Read the model definition and answer for the solid it produces. Units are mm, in the model's axes. A direction names the side the tool comes from. Round coordinates to 2 decimals unless told otherwise and drop trailing zeros. Loops run counter-clockwise (first coordinate to the right, second up) from the corner with the lowest first, then second, coordinate; pieces in that order, holes last. Notation, with made-up numbers: (3.5, -2) -> (13.5, -2) arc R21 ccw to (13.5, 21) -> close; hole circle Ø10 at (57.5, -0.5). An arc over 180 degrees is marked (long way). Put each result on its own line as item: value.
from build123d import *

# Parameters (mm, degrees)
SKETCH_1_R          = 0.9
SKETCH_1_R_2        = 0.8
EXTRUDE_1_DEPTH     = 3.2
EXTRUDE_1_2_DEPTH   = 3.2
SKETCH_2_W          = 51.115590172
SKETCH_2_H          = 4.08
EXTRUDE_2_DEPTH     = 1.2
EXTRUDE_START       = -3.2
EXTRUDE_3_DEPTH     = 3.2
SKETCH_4_R          = 2
CUT_EXTRUDE_1_DEPTH = 2
FILLET_1_R          = 0.5


with BuildPart() as part:
    # Sketch 1 → Extrude 1 (new body)
    with BuildSketch(Plane.XY):
        with BuildLine():
            Line((-32.44, 5.005), (-31.75, 5.005))
            ThreePointArc((-31.75, 5.005), (-31.624500996, 4.977488532), (-31.522019738, 4.9))
            Line((-31.522019738, 4.9), (-28, 4.9))
            Line((-28, 4.9), (-28, 6.996662954))
            ThreePointArc((-28, 6.996662954), (-27.853553391, 7.350216345), (-27.5, 7.496662954))
            Line((-27.5, 7.496662954), (-22.181386307, 7.496662954))
            Line((-22.181386307, 7.496662954), (-22.181386307, 9.626936565))
            ThreePointArc((-22.181386307, 9.626936565), (-22.687871835, 9.843944297), (-23.142051903, 10.155938547))
            Line((-23.142051903, 10.155938547), (-24.268653026, 11.105751817))
            ThreePointArc((-24.268653026, 11.105751817), (-24.871565433, 11.455249887), (-25.557795086, 11.576662954))
            Line((-25.557795086, 11.576662954), (-30.347104952, 11.576662954))
            ThreePointArc((-30.347104952, 11.576662954), (-31.033334605, 11.455249887), (-31.636247011, 11.105751817))
            Line((-31.636247011, 11.105751817), (-32.42914206, 10.437278989))
            ThreePointArc((-32.42914206, 10.437278989), (-32.9535992, 9.751314044), (-33.14, 8.908190127))
            Line((-33.14, 8.908190127), (-33.14, 5.705))
            ThreePointArc((-33.14, 5.705), (-32.934974747, 5.210025253), (-32.44, 5.005))
        make_face()
        with Locations(Location((-27.952450019, 9.676662954, 0), (0, 0, 270))):
            Circle(SKETCH_1_R, mode=Mode.SUBTRACT)
        with Locations(Location((-31.24, 6.905, 0), (0, 0, 270))):
            Circle(SKETCH_1_R_2, mode=Mode.SUBTRACT)
    extrude(amount=EXTRUDE_1_DEPTH)



with BuildPart() as body_2:
    # Sketch 1 → Extrude 1 2 (new body)
    with BuildSketch(Plane.XY):
        with BuildLine():
            Line((28, 6.996662954), (28, 4.9))
            Line((28, 4.9), (31.522019738, 4.9))
            ThreePointArc((31.522019738, 4.9), (31.624500996, 4.977488532), (31.75, 5.005))
            Line((31.75, 5.005), (32.44, 5.005))
            ThreePointArc((32.44, 5.005), (32.934974747, 5.210025253), (33.14, 5.705))
            Line((33.14, 5.705), (33.14, 8.908190127))
            ThreePointArc((33.14, 8.908190127), (32.9535992, 9.751314044), (32.42914206, 10.437278989))
            Line((32.42914206, 10.437278989), (31.636247011, 11.105751817))
            ThreePointArc((31.636247011, 11.105751817), (31.033334605, 11.455249887), (30.347104952, 11.576662954))
            Line((30.347104952, 11.576662954), (25.557795086, 11.576662954))
            ThreePointArc((25.557795086, 11.576662954), (24.871565433, 11.455249887), (24.268653026, 11.105751817))
            Line((24.268653026, 11.105751817), (23.142051903, 10.155938547))
            ThreePointArc((23.142051903, 10.155938547), (22.687871835, 9.843944297), (22.181386307, 9.626936565))
            Line((22.181386307, 9.626936565), (22.181386307, 7.496662954))
            Line((22.181386307, 7.496662954), (27.5, 7.496662954))
            ThreePointArc((27.5, 7.496662954), (27.853553391, 7.350216345), (28, 6.996662954))
        make_face()
        with Locations(Location((27.952450019, 9.676662954, 0), (0, 0, 270))):
            Circle(SKETCH_1_R, mode=Mode.SUBTRACT)
        with Locations(Location((31.24, 6.905, 0), (0, 0, 270))):
            Circle(SKETCH_1_R_2, mode=Mode.SUBTRACT)
    extrude(amount=EXTRUDE_1_2_DEPTH)


with BuildPart() as part_1:
    add(part.part)

    add(body_2.part)  # Extrude 2 merges body 2
    # Sketch 2 → Extrude 2 (add)
    with BuildSketch(Plane.XY.offset(3.2)):
        with Locations((0, 9.536662954)):
            Rectangle(SKETCH_2_W, SKETCH_2_H)
    extrude(amount=-EXTRUDE_2_DEPTH)

    # Sketch 3 → Extrude 3 (add)
    with BuildSketch(Plane.XY.offset(3.2).offset(EXTRUDE_START)):
        with BuildLine():
            Line((46.240904424, 11.074408529), (31.674834812, 11.073219269))
            Line((31.674834812, 11.073219269), (32.42914206, 10.437278989))
            ThreePointArc((32.42914206, 10.437278989), (32.9535992, 9.751314044), (33.14, 8.908190127))
            Line((33.14, 8.908190127), (33.14, 5.705))
            ThreePointArc((33.14, 5.705), (33.130629249, 5.59084554), (33.102767884, 5.479747403))
            Line((33.102767884, 5.479747403), (47.600381988, 5.480931075))
            ThreePointArc((47.600381988, 5.480931075), (50.358005162, 6.623439781), (51.500063555, 9.381249481))
            Line((51.500063555, 9.381249481), (51.497785633, 37.281249388))
            ThreePointArc((51.497785633, 37.281249388), (50.355276927, 40.038872563), (47.597467227, 41.180930956))
            Line((47.597467227, 41.180930956), (-47.402532456, 41.17317459))
            ThreePointArc((-47.402532456, 41.17317459), (-50.160155631, 40.030665884), (-51.302214024, 37.272856184))
            Line((-51.302214024, 37.272856184), (-51.299936102, 9.372856277))
            ThreePointArc((-51.299936102, 9.372856277), (-50.157427396, 6.615233102), (-47.399617696, 5.473174709))
            Line((-47.399617696, 5.473174709), (-33.10090616, 5.474342141))
            ThreePointArc((-33.10090616, 5.474342141), (-33.130157341, 5.58802631), (-33.14, 5.705))
            Line((-33.14, 5.705), (-33.14, 8.908190127))
            ThreePointArc((-33.14, 8.908190127), (-32.9535992, 9.751314044), (-32.42914206, 10.437278989))
            Line((-32.42914206, 10.437278989), (-31.673318835, 11.074497357))
            Line((-31.673318835, 11.074497357), (-46.40016763, 11.073294969))
            ThreePointArc((-46.40016763, 11.073294969), (-48.972219468, 12.138427704), (-50.037772184, 14.71030558))
            Line((-50.037772184, 14.71030558), (-50.039543904, 36.410348688))
            ThreePointArc((-50.039543904, 36.410348688), (-48.974411169, 38.982400526), (-46.402533293, 40.047953242))
            Line((-46.402533293, 40.047953242), (46.597651817, 40.055546331))
            ThreePointArc((46.597651817, 40.055546331), (49.169703655, 38.990413596), (50.235256371, 36.41853572))
            Line((50.235256371, 36.41853572), (50.237028092, 14.718492612))
            ThreePointArc((50.237028092, 14.718492612), (49.171895357, 12.146440774), (46.600017481, 11.080888058))
            ThreePointArc((46.600017481, 11.080888058), (46.420490045, 11.076035874), (46.240904424, 11.074408529))
        make_face()
    extrude(amount=EXTRUDE_3_DEPTH)

    # Sketch 4 → Cut-Extrude 1 (cut)
    with BuildSketch(Plane.XY.offset(3.2)):
        with Locations((-27.952450019, 9.676662954)):
            Circle(SKETCH_4_R)
        with Locations((27.952450019, 9.676662954)):
            Circle(SKETCH_4_R)
        with Locations((-31.24, 6.905)):
            Circle(SKETCH_4_R)
        with Locations((31.24, 6.905)):
            Circle(SKETCH_4_R)
    extrude(amount=-CUT_EXTRUDE_1_DEPTH, mode=Mode.SUBTRACT)

    # Fillet 1
    fillet_1_edges = [part_1.edges().sort_by_distance(p)[0] for p in [
        (-27.327950219, 11.576662954, 2.2),
        (-28.576949819, 11.576662954, 2.2),
        (28.576949819, 11.576662954, 2.2),
        (27.327950219, 11.576662954, 2.2),
    ]]
    fillet(fillet_1_edges, radius=FILLET_1_R)


solid = part_1.part
Item 1: The part is cut by section B-B (x = 3.5). Determine the outline of the cut face in (y, z), then the cut area to 3 significant figures.
Derived:
outline: (7.5, 2) -> (11.58, 2) -> (11.58, 3.2) -> (7.5, 3.2) -> close; (40.05, 0) -> (41.18, 0) -> (41.18, 3.2) -> (40.05, 3.2) -> close
area: 8.50 mm^2
Item 2: For a pull along Y with two mould halves and no side action, classify faces 1 (the flat face through (28, 6, 2)), 2 (the cylindrical face through (50.385, 40.008, 1.578)), 3 (the cylindrical face through (-48.944, 12.11, 1.578)), 4 (the flat face through (30, 4.9, 2)) as pulls with the +Y half, pulls with the -Y half, needs draft (parallel to the pull), parting line crosses it, or undercut.
Derived:
face 1: needs draft
face 2: pulls with the +Y half
face 3: undercut
face 4: pulls with the -Y half
Item 3: Flat-ended cylindrical pins translate along their axes: pin 1 Ø2 at (x, y) = (-28, 9) entering from +Z; pin 2 Ø1.4 at (x, y) = (27.95, 9.68) entering from -Z; pin 3 Ø1.2 at (x, y) = (11.5, 9) entering from -Z; pin 4 Ø1 at (y, z) = (8, 1.5) entering from +X. Find the tip coordinate at first contact, or state that the pin passes through.
Derived:
pin 1: stops at z = 1.2
pin 2: passes through
pin 3: stops at z = 2
pin 4: stops at x = 51.4
Item 4: The part is cut by section A-A (y = 12.5). Determine the outline of the cut face in (x, z), then the cut area to 3 significant figures.
Derived:
outline: (-51.3, 0) -> (-49.29, 0) -> (-49.29, 3.2) -> (-51.3, 3.2) -> close; (49.48, 0) -> (51.5, 0) -> (51.5, 3.2) -> (49.48, 3.2) -> close
area: 12.9 mm^2
Item 5: Which of the six approach directions +Z, -Z, +X, -X, +Y, -Y give full straight-line access (tool end or side, diameter ignored) to faces 5 (the cylindrical face through (-50.13, 40.06, 1.58)), 6 (the cylindrical face through (-49.003, 38.954, 1.578)), 7 (the flat face through (-30, 7, 1.2))?
Derived:
face 5: +Z, -Z, -X, +Y
face 6: +Z, -Z
face 7: +Z
Item 6: Find the intervals of material crossed by line 1 along Y through (x, z) = (-5, 2.25); line 2 along X through (y, z) = (18, 2.6); line 3 along Y through (x, z) = (-30, 2.1), in increasing order.
Derived:
line 1: y = 7.5 to 11.58, 40.05 to 41.18
line 2: x = -51.3 to -50.04, 50.24 to 51.5
line 3: y = 4.9 to 5.34, 8.47 to 11.58, 40.05 to 41.17
